Work out the finished part from the listing and answer in its coordinate system (mm). Face numbers are marked on the shaded views. A direction names the side the tool comes from. Coordinates: 2 decimals unless noted, no trailing zeros. Order: outer loops, then holes, each group sorted by start corner. A loop starts at its lowest first (then second) coordinate and runs counter-clockwise, first axis right, second up. Notation, with made-up numbers: M 51,28.25 L 106,28.25 A26 ccw 106,66.25 Z; hole C 78.5,15 d11. An arc over 180 degrees is marked long. Write item = value, one per line. Start each with the question number.
Q1. A tool of negligible diameter and unlimited length cuts with its end or side. For the marked faces 4 and 5, from which of +Z, -Z, +X, -X, +Y, -Y can it reach the whole face along a straight path? Write none if from no direction.
Q2. Determine the mould class of the marked faces 1, 2 and 3 for opening direction Y: released by +Y, released by -Y, zero draft, split by the parting line, or undercut.
Q3. Find section D-D on x = 17. Give the vertices of the cut face in (y, z) (3 decimals), and give its area (3 significant figures).
Q4. Find section A-A on x = 28. Give the vertices of the cut face in (y, z) (3 decimals), and give its area (3 significant figures).
Q5. Straight lines are drawn through the part: line 1 along Y through (x, z) = (46, 18.5); line 2 along Y through (x, z) = (47, 3.5); line 3 along X through (y, z) = (25, 2). For each, find the intervals that lie inside material, in ascending order.
Q6. Each of these flat-tipped pins is pushed along its axis until it touches: P1, Ø20.5, axis at x = 28.575, y = 25.4, coming from the +Z side (3 decimals); P2, Ø5, axis at y = 5.5, z = 37.5, coming from the -X side; P3, Ø3.5, axis at y = 25.4, z = 4.76, coming from the -X side; P4, Ø2.5, axis at y = 25.4, z = 4.76, coming from the +X side. Where does it stop, or does it pass through?
Q7. Find section B-B on z = 11. Give the number of separate pieces and of enclosed holes in the cut face, and give its area (3 significant figures).
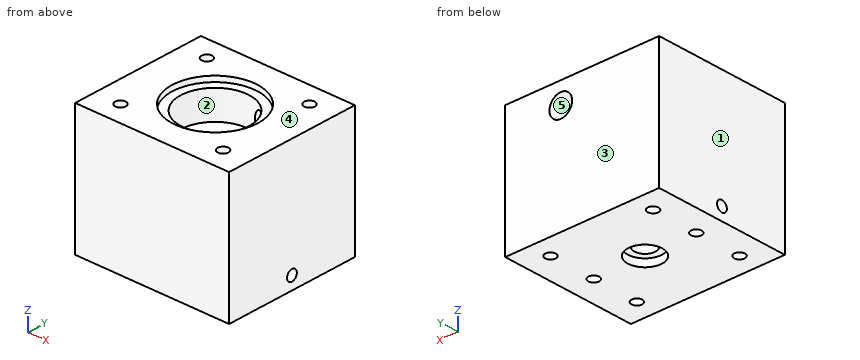
```python
from build123d import *

# Parameters (mm, degrees)
SKETCH1_W           = 57.15
SKETCH1_H           = 50.8
BOSS_EXTRUDE1_DEPTH = 47.625
SKETCH2_R           = 3.8354
CUT_EXTRUDE1_DEPTH  = 91.08275709
SKETCH3_R           = 12.7
CUT_EXTRUDE2_DEPTH  = 12.7
SKETCH4_R           = 15.875
CUT_EXTRUDE3_DEPTH  = 2.032
SKETCH5_R           = 4.2164
CUT_EXTRUDE4_DEPTH  = 25.4
SKETCH6_R           = 6.35
CUT_EXTRUDE5_DEPTH  = 2.794
SKETCH7_R           = 1.98501
CUT_EXTRUDE6_DEPTH  = 6.35
SKETCH8_R           = 1.98501
CUT_EXTRUDE7_DEPTH  = 91.082757147
SKETCH9_R           = 1.98501
CUT_EXTRUDE9_DEPTH  = 11.1125
CUT_EXTRUDE10_START = -11.1125
SKETCH10_R          = 1.98501
CUT_EXTRUDE10_DEPTH = 11.1125


with BuildPart() as part:
    # Sketch1 → Boss-Extrude1 (new body)
    with BuildSketch(Plane.XY):
        with Locations((28.575, 25.4)):
            Rectangle(SKETCH1_W, SKETCH1_H)
    extrude(amount=BOSS_EXTRUDE1_DEPTH)

    # Sketch2 → Cut-Extrude1 (cut, through all)
    with BuildSketch(Plane.XY.offset(47.625)):
        with Locations((28.575, 25.4)):
            Circle(SKETCH2_R)
    extrude(amount=-CUT_EXTRUDE1_DEPTH, mode=Mode.SUBTRACT)

    # Sketch3 → Cut-Extrude2 (cut)
    with BuildSketch(Plane.XY.offset(47.625)):
        with Locations((28.575, 25.4)):
            Circle(SKETCH3_R)
    extrude(amount=-CUT_EXTRUDE2_DEPTH, mode=Mode.SUBTRACT)

    # Sketch4 → Cut-Extrude3 (cut)
    with BuildSketch(Plane.XY.offset(47.625)):
        with Locations((28.575, 25.4)):
            Circle(SKETCH4_R)
    extrude(amount=-CUT_EXTRUDE3_DEPTH, mode=Mode.SUBTRACT)

    # Sketch5 → Cut-Extrude4 (cut)
    with BuildSketch(Plane(origin=(0, 50.8, 0), x_dir=(1, 0, 0), z_dir=(0, 1, 0))):
        with Locations(Location((36.5125, -39.6875, 0), (0, 0, 270))):
            Circle(SKETCH5_R)
    extrude(amount=-CUT_EXTRUDE4_DEPTH, mode=Mode.SUBTRACT)

    # Sketch6 → Cut-Extrude5 (cut)
    with BuildSketch(Plane(origin=(0, 0, 0), x_dir=(-1, 0, 0), z_dir=(0, 0, -1))):
        with Locations((-28.575, 25.4)):
            Circle(SKETCH6_R)
    extrude(amount=-CUT_EXTRUDE5_DEPTH, mode=Mode.SUBTRACT)

    # Sketch7 → Cut-Extrude6 (cut)
    with BuildSketch(Plane(origin=(0, 0, 0), x_dir=(-1, 0, 0), z_dir=(0, 0, -1))):
        with Locations((-9.525, 25.4)):
            Circle(SKETCH7_R)
        with Locations((-47.625, 25.4)):
            Circle(SKETCH7_R)
    extrude(amount=-CUT_EXTRUDE6_DEPTH, mode=Mode.SUBTRACT)

    # Sketch8 → Cut-Extrude7 (cut, through all)
    with BuildSketch(Plane(origin=(0, 0, 0), x_dir=(-1, 0, 0), z_dir=(0, 0, -1))):
        with Locations((-47.625, 42.8625)):
            Circle(SKETCH8_R)
        with Locations((-9.525, 42.8625)):
            Circle(SKETCH8_R)
        with Locations((-9.525, 7.9375)):
            Circle(SKETCH8_R)
        with Locations((-47.625, 7.9375)):
            Circle(SKETCH8_R)
    extrude(amount=-CUT_EXTRUDE7_DEPTH, mode=Mode.SUBTRACT)

    # Sketch9 → Cut-Extrude9 (cut)
    with BuildSketch(Plane.ZY):
        with Locations((4.7625, 25.4)):
            Circle(SKETCH9_R)
    extrude(amount=-CUT_EXTRUDE9_DEPTH, mode=Mode.SUBTRACT)

    # Sketch10 → Cut-Extrude10 (cut)
    with BuildSketch(Plane(origin=(57.15, 0, 0), x_dir=(0, 0, -1), z_dir=(1, 0, 0)).offset(CUT_EXTRUDE10_START)):
        with Locations(Location((-4.7625, 25.4, 0), (0, 0, 180))):
            Circle(SKETCH10_R)
    extrude(amount=CUT_EXTRUDE10_DEPTH, mode=Mode.SUBTRACT)


solid = part.part
```
Findings below:
q1.face_4 = +Z, +X, -X, +Y, -Y
q1.face_5 = +Y
q2.face_1 = zero draft
q2.face_2 = undercut
q2.face_3 = released by +Y
q3.outline = M 0,0 L 50.8,0 L 50.8,47.625 L 36.264,47.625 L 36.264,45.593 L 30.626,45.593 L 30.626,34.925 L 20.174,34.925 L 20.174,45.593 L 14.536,45.593 L 14.536,47.625 L 0,47.625 Z
q3.area = 2,260 mm^2
q4.outline = M 0,0 L 19.076,0 L 19.076,2.794 L 21.608,2.794 L 21.608,34.925 L 12.713,34.925 L 12.713,45.593 L 9.535,45.593 L 9.535,47.625 L 0,47.625 Z; M 29.192,2.794 L 31.724,2.794 L 31.724,0 L 50.8,0 L 50.8,47.625 L 41.265,47.625 L 41.265,45.593 L 38.087,45.593 L 38.087,34.925 L 29.192,34.925 Z
q4.area = 1,810 mm^2
q5.line_1 = 0 to 6.8, 9.08 to 41.72, 44 to 50.8
q5.line_2 = 0 to 6.05, 9.82 to 23.52, 27.28 to 40.98, 44.75 to 50.8
q5.line_3 = 0 to 7.58, 11.47 to 22.24, 34.91 to 45.68, 49.57 to 57.15
q6.P1 = 34.925
q6.P2 = 0
q6.P3 = 11.11
q6.P4 = 46.04
q7.separate_pieces = 1
q7.enclosed_holes = 5
q7.area = 2,810 mm^2
